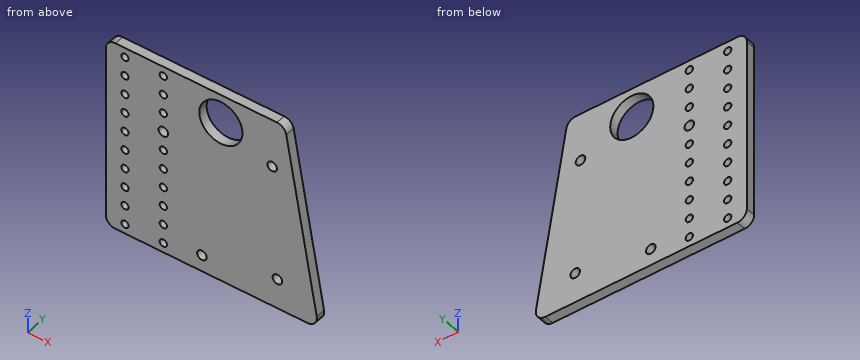
from build123d import *

# Parameters (mm, degrees)
INITIAL_PLATE_DEPTH         = 6.35
SKETCH3_R                   = 2.413
INITIAL_MOUNTING_HOLE_DEPTH = 7.35
MOUNTING_PATTERN_COUNT      = 10
MOUNTING_PATTERN_PITCH      = 12.7
SKETCH2_R                   = 3.175
BEARING_STACK_HOLES_DEPTH   = 7.35
FILLET1_R                   = 6.35
SKETCH4_R                   = 14.2875
CUT_EXTRUDE1_DEPTH          = 7.35


with BuildPart() as part:
    # Sketch1 → Initial Plate (new body)
    with BuildSketch(Plane(origin=(0, 0, 0), x_dir=(1, 0, 0), z_dir=(0, 1, 0))):
        Polygon((-64.403593083, -58.02125503), (54.172880367, -58.02125503), (76.566406917, 68.97874497), (-64.403593083, 68.97874497), align=None)
    extrude(amount=INITIAL_PLATE_DEPTH)

    # Sketch3 → Initial Mounting Hole (cut, through all)
    with BuildSketch(Plane(origin=(0, 6.35, 0), x_dir=(1, 0, 0), z_dir=(0, 1, 0))):
        with Locations((-51.703593083, -51.67125503)):
            Circle(SKETCH3_R)
        with Locations((-26.303593083, -51.67125503)):
            Circle(SKETCH3_R)
    initial_mounting_hole = extrude(amount=-INITIAL_MOUNTING_HOLE_DEPTH, mode=Mode.SUBTRACT)

    # Mounting Pattern: Initial Mounting Hole ×10
    with Locations(*[(0, 0, -i * MOUNTING_PATTERN_PITCH) for i in range(1, MOUNTING_PATTERN_COUNT)]):
        add(initial_mounting_hole, mode=Mode.SUBTRACT)

    # Sketch2 → Bearing Stack Holes (cut, through all)
    with BuildSketch(Plane(origin=(0, 6.35, 0), x_dir=(1, 0, 0), z_dir=(0, 1, 0))):
        with Locations((-26.303593083, -13.57125503)):
            Circle(SKETCH2_R)
        with Locations((49.243157186, 49.193730621)):
            Circle(SKETCH2_R)
        with Locations((45.737063665, -26.273966523)):
            Circle(SKETCH2_R)
        with Locations((-0.785076667, 58.015058047)):
            Circle(SKETCH2_R)
    extrude(amount=-BEARING_STACK_HOLES_DEPTH, mode=Mode.SUBTRACT)

    # Fillet1
    fillet1_edges = [part.edges().sort_by_distance(p)[0] for p in [
        (54.172880367, 3.175, 58.02125503),
        (-64.403593083, 3.175, 58.02125503),
        (-64.403593083, 3.175, -68.97874497),
        (76.566406917, 3.175, -68.97874497),
    ]]
    fillet(fillet1_edges, radius=FILLET1_R)

    # Sketch4 → Cut-Extrude1 (cut, through all)
    with BuildSketch(Plane(origin=(0, 6.35, 0), x_dir=(1, 0, 0), z_dir=(0, 1, 0))):
        with Locations((11.792603678, -38.977523898)):
            Circle(SKETCH4_R)
    extrude(amount=-CUT_EXTRUDE1_DEPTH, mode=Mode.SUBTRACT)


solid = part.part
Source: CAD feature listing. Evaluate the final solid. Frame: model axes, mm. Round coordinates to 2 decimals unless told otherwise and drop trailing zeros. Loops run counter-clockwise (first coordinate to the right, second up) from the corner with the lowest first, then second, coordinate; pieces in that order, holes last.
Q1. First-contact query: P1, Ø1.5, axis at y = 2, z = 2.5, coming from the +X side (3 decimals); P2, Ø3, axis at x = -51.7, z = -49.93, coming from the +Y side; P3, Ø2, axis at y = 3.5, z = -51, coming from the +X side. Flat tips, straight axial feed; report the tip coordinate or a pass-through.
Q2. Ray query, line 1 (X direction, y = 2.5, z = -1); line 2 (X direction, y = 1, z = -62); line 3 (X direction, y = 3, z = 41). Return the intervals inside material, ascending.
Q3. Section B-B, the plane y = 2. State how many separate pieces and enclosed holes the cut face has, plus the area to 3 significant figures.
Q4. Section C-C, the plane z = -29. Return loops of the section in (x, y).
Q5. Section A-A, the plane x = 23. Return loops of the section in (y, z).
Solutions:
1. P1: stops at x = 64.095
1. P2: passes through
1. P3: stops at x = 73.57
2. line 1: x = -64.4 to -53.23, -50.18 to -27.83, -24.78 to 64.58
2. line 2: x = -64.4 to -54.03, -49.37 to -28.63, -23.97 to 75.32
2. line 3: x = -64.4 to -53.01, -50.4 to -27.61, -25 to -2.35, 25.94 to 57.17
3. separate pieces: 1
3. enclosed holes: 24
3. area: 15,300 mm2
4. outline: (-64.4, 0) - (69.52, 0) - (69.52, 6.35) - (-64.4, 6.35) - close
5. outline: (0, -68.98) - (6.35, -68.98) - (6.35, 30.12) - (0, 30.12) - close; (0, 47.84) - (6.35, 47.84) - (6.35, 58.02) - (0, 58.02) - close
